The model under review builds one solid part; all positions refer to its coordinate system, in mm. Face numbers are marked on the shaded views. Coordinates: 2 decimals unless noted, no trailing zeros. Order: outer loops, then holes, each group sorted by start corner. A loop starts at its lowest first (then second) coordinate and runs counter-clockwise, first axis right, second up. Notation, with made-up numbers: M -35,-0.5 L 15,-0.5 A12 ccw 15,6.5 Z; hole C -27.75,4 d5. An arc over 180 degrees is marked long. Write each question's results on one line, items separated by ' | '.
from build123d import *

# Parameters (mm, degrees)
SKETCH_1_R      = 3.05
EXTRUDE_1_DEPTH = 3
FILLET_1_R      = 0.5


with BuildPart() as part:
    # 草图1 → 凸台-拉伸1 (new body)
    with BuildSketch(Plane(origin=(0, 0, 0), x_dir=(1, 0, 0), z_dir=(0, 1, 0))):
        with BuildLine():
            Line((0, 0), (23.75, 0))
            ThreePointArc((23.75, 0), (30, 6.25), (23.75, 12.5))
            Line((23.75, 12.5), (0, 12.5))
            Line((0, 12.5), (0, 0))
        make_face()
        with Locations(Location((23.75, 6.25, 0), (0, 0, 270))):
            Circle(SKETCH_1_R, mode=Mode.SUBTRACT)
    extrude(amount=EXTRUDE_1_DEPTH)

    # 圆角1
    fillet_1_edges = [part.edges().sort_by_distance(p)[0] for p in [
        (23.75, 0, -9.3),
        (23.75, 3, -9.3),
        (30, 3, -6.25),
        (11.875, 3, -12.5),
        (0, 3, -6.25),
        (11.875, 0, -12.5),
        (30, 0, -6.25),
        (11.875, 0, 0),
        (0, 0, -6.25),
        (0, 1.5, -12.5),
        (0, 1.5, 0),
        (11.875, 3, 0),
    ]]
    fillet(fillet_1_edges, radius=FILLET_1_R)


solid = part.part
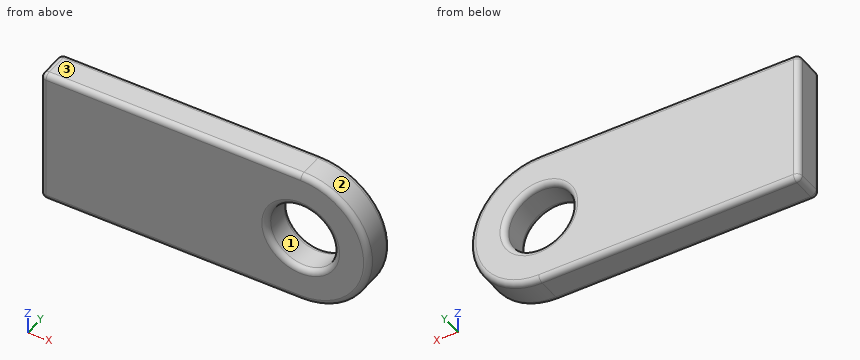
1) To check wall thickness, follow line 1 along X through (y, z) = (1.3, -6.25); line 2 along X through (y, z) = (0.95, -8.75); line 3 along Z through (x, y) = (10, 2.65). State the ranges of each line that lie inside material, in increasing order.
Solutions:
line 1: 0 to 20.7, 26.8 to 30 | line 2: 0 to 22, 25.5 to 29.48 | line 3: -12.48 to -0.02
2) Take a section at B-B on y = 1.75. State the section outline as (x, z) points.
Solutions:
outline: M 0,-12 A0.5 ccw 0.5,-12.5 L 23.75,-12.5 A6.25 ccw 23.75,0 L 0.5,0 A0.5 ccw 0,-0.5 Z; hole C 23.75,-6.25 d6.1
3) For pin 1 (6 mm diameter, centred on x = 26.5, z = -8, fed in from -Y); pin 2 (3.5 mm diameter, centred on x = 23.75, z = -6.25, fed in from -Y), all flat-tipped, find the tip position at first contact; note any pin that passes through.
Solutions:
pin 1: y = 0 | pin 2: through
4) The part is to be moulded in two halves that separate along X. For the marked faces 1, 2 and 3, say which applies: pulls with the +X half, pulls with the -X half, needs draft (parallel to the pull), parting line crosses it, or undercut.
Solutions:
face 1: undercut | face 2: pulls with the +X half | face 3: needs draft
5) Take a section at A-A on z = -6.25. State the section outline as (x, y) points, plus the area to 3 significant figures.
Solutions:
outline: M 0,0.5 A0.5 ccw 0.5,0 L 20.2,0 A0.5 ccw 20.7,0.5 L 20.7,2.5 A0.5 ccw 20.2,3 L 0.5,3 A0.5 ccw 0,2.5 Z; M 26.8,0.5 A0.5 ccw 27.3,0 L 29.5,0 A0.5 ccw 30,0.5 L 30,2.5 A0.5 ccw 29.5,3 L 27.3,3 A0.5 ccw 26.8,2.5 Z | area: 71.3 mm2
